Work out the finished part from the listing and answer in its coordinate system (mm). Give positions to 0.01 mm unless a question says otherwise; leave off trailing zeros. Write each loop counter-clockwise with the first axis right and the second up, starting at its lowest first coordinate (ties: lowest second). Pieces come first, ordered by that corner, then holes. Notation, with made-up numbers: (75, 49) -> (122, 49) arc R10 ccw to (122, 58) -> close; hole circle Ø9 at (5, 80.5). An arc over 180 degrees is marked (long way). Use a Markdown table: item, result. Add a question column.
Q1. Consider line 1 (Y direction, x = 48, z = 0.45); line 2 (X direction, y = 32.5, z = 1.65). Determine where each line is inside the solid, lowest interval first.
Q2. Section B-B, the plane y = 33 is taken. Give the vertices of the cut face in (x, z).
Q3. For a pull along X with two mould halves and no side action, classify faces 1 (the face through (-49.86, 33.59, 0.84)), 2 (the face through (-51.64, -36.6, 0.86)), 3 (the face through (-1, 1, 1.7)) as pulls with the +X half, pulls with the -X half, needs draft (parallel to the pull), parting line crosses it, or undercut.
Q4. Section A-A, the plane x = -48 is taken. Give the vertices of the cut face in (y, z).
from build123d import *

# Parameters (mm, degrees)
ESQUISSE1_W                     = 105
ESQUISSE1_H                     = 75
BOSS_EXTRU_1_DEPTH              = 1.7
D_GAGEMENT_M3_51_D              = 3.9
R_P_TITION_LIN_AIRE1_COUNT      = 2
R_P_TITION_LIN_AIRE1_PITCH      = 96
R_P_TITION_LIN_AIRE1_COUNT_DIR2 = 2
R_P_TITION_LIN_AIRE1_PITCH_DIR2 = 66
CONG_1_R                        = 3


with BuildPart() as part:
    # Esquisse1 → Boss.-Extru.1 (new body)
    with BuildSketch(Plane.XY):
        Rectangle(ESQUISSE1_W, ESQUISSE1_H)
    extrude(amount=BOSS_EXTRU_1_DEPTH)

    # Dégagement M3.51 (through all)
    with Locations(Plane.XY.offset(1.7)):
        with Locations((48, 33)):
            d_gagement_m3_51 = Hole(D_GAGEMENT_M3_51_D / 2)

    # Répétition linéaire1: D_gagement M3.51 2 × 2
    with Locations(*[(-i * R_P_TITION_LIN_AIRE1_PITCH, -j * R_P_TITION_LIN_AIRE1_PITCH_DIR2, 0) for i in range(R_P_TITION_LIN_AIRE1_COUNT) for j in range(R_P_TITION_LIN_AIRE1_COUNT_DIR2) if (i, j) != (0, 0)]):
        add(d_gagement_m3_51, mode=Mode.SUBTRACT)

    # Congé1
    cong_1_edges = [part.edges().sort_by_distance(p)[0] for p in [
        (52.5, -37.5, 0.85),
        (52.5, 37.5, 0.85),
        (-52.5, 37.5, 0.85),
        (-52.5, -37.5, 0.85),
    ]]
    fillet(cong_1_edges, radius=CONG_1_R)


solid = part.part
Result set:
| question | item | result |
|---|---|---|
| 1 | line 1 | y = -37.5 to -34.95, -31.05 to 31.05, 34.95 to 37.5 |
| 1 | line 2 | x = -52.5 to -49.88, -46.12 to 46.12, 49.88 to 52.5 |
| 2 | outline | (-52.5, 0) -> (-49.95, 0) -> (-49.95, 1.7) -> (-52.5, 1.7) -> close; (-46.05, 0) -> (46.05, 0) -> (46.05, 1.7) -> (-46.05, 1.7) -> close; (49.95, 0) -> (52.5, 0) -> (52.5, 1.7) -> (49.95, 1.7) -> close |
| 3 | face 1 | undercut |
| 3 | face 2 | pulls with the -X half |
| 3 | face 3 | needs draft |
| 4 | outline | (-37.5, 0) -> (-34.95, 0) -> (-34.95, 1.7) -> (-37.5, 1.7) -> close; (-31.05, 0) -> (31.05, 0) -> (31.05, 1.7) -> (-31.05, 1.7) -> close; (34.95, 0) -> (37.5, 0) -> (37.5, 1.7) -> (34.95, 1.7) -> close |
